Answer from the drawing. Dimensions are ordinates in mm from the lowest x, y and z of the part. A direction names the side the tool comes from. Round coordinates to 2 decimals unless told otherwise and drop trailing zeros. Write each loop counter-clockwise with the first axis right and the second up, starting at its lowest first coordinate (ties: lowest second). Pieces come first, ordered by that corner, then holes.
1. Straight lines are drawn through the part: probe 1 along Y at (x, z) = (7.25, 13); probe 2 along Z at (x, y) = (10.5, 14.5); probe 3 along Y at (x, z) = (10.5, 5). For each, find the intervals that lie inside material, in ascending order.
2. Determine the mould class of the marked faces 3, 4 and 5 for opening direction Z: pulls with the +Z half, pulls with the -Z half, needs draft (parallel to the pull), parting line crosses it, or undercut.
3. Find section A-A (y = 8.25). Write down the section's boundary in (x, z).
4. A tool of negligible diameter and unlimited length cuts with its end or side. For the marked faces 1 and 2, from which of +Z, -Z, +X, -X, +Y, -Y can it reach the whole face along a straight path? Write none if from no direction.
5. Flat-ended cylindrical pins translate along their axes: pin 1 Ø6 at (x, y) = (7.5, 15) entering from -Z; pin 2 Ø4 at (x, y) = (5, 15) entering from -Z; pin 3 Ø0.5 at (x, y) = (7, 24) entering from +Z. Find the tip coordinate at first contact, or state that the pin passes through.
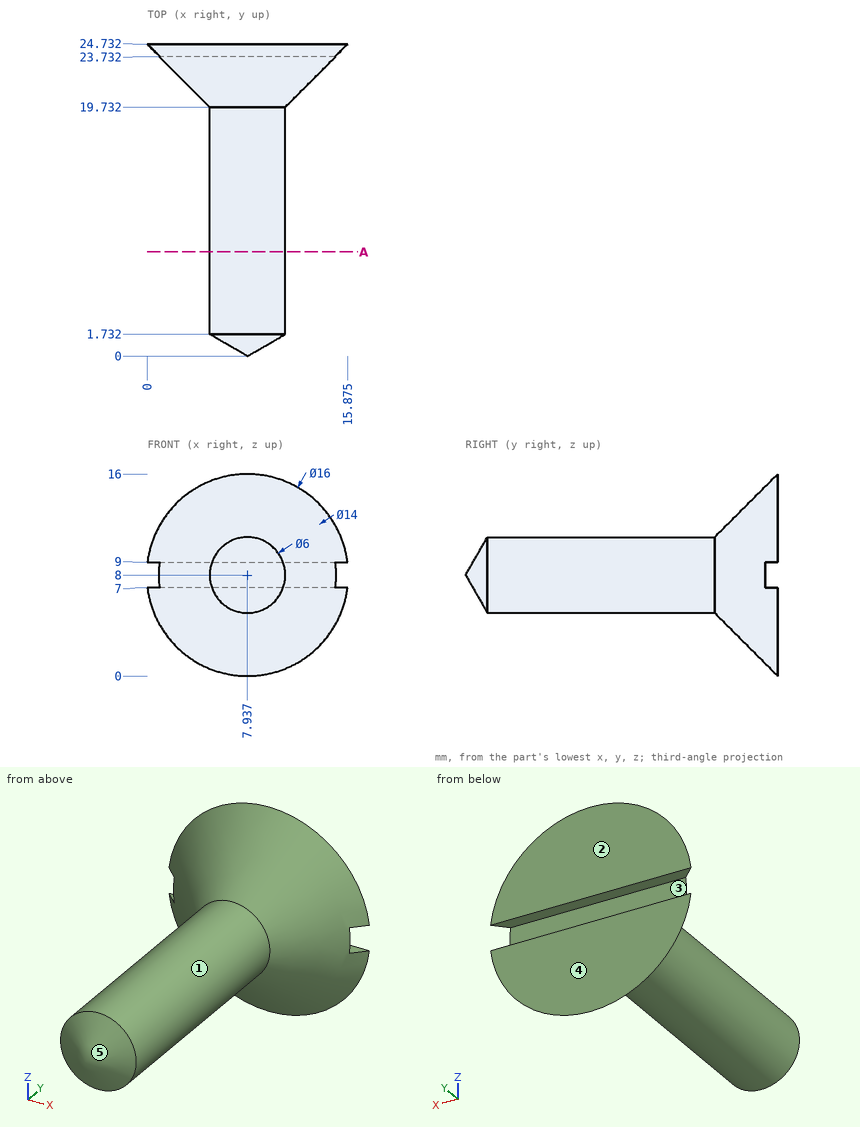
Worked answers:
1. probe 1: y = 21.78 to 24.73
1. probe 2: z = 6.44 to 9.56
1. probe 3: y = 20.68 to 24.73
2. face 3: undercut
2. face 4: needs draft
2. face 5: parting line crosses it
3. outline: circle Ø6 at (7.94, 8)
4. face 1: -Y
4. face 2: +Z, -Z, +X, -X, +Y
5. pin 1: stops at z = 5
5. pin 2: stops at z = 5.15
5. pin 3: stops at z = 15.46
